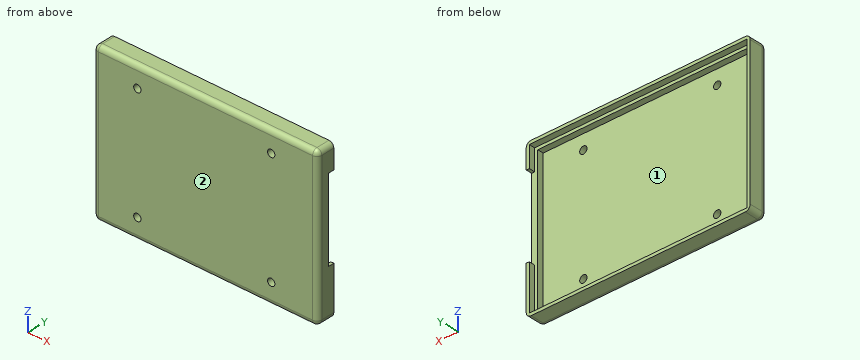
Autodesk Inventor part; units mm, degrees
ref_plane "YZ Plane" through (0, 0, 0) normal (1, 0, 0) x (0, 1, 0)
ref_plane "XZ Plane" through (0, 0, 0) normal (0, 1, 0) x (-1, 0, 0)
ref_plane "XY Plane" through (0, 0, 0) normal (0, 0, 1) x (1, 0, 0)
sketch "Sketch1" plane through (0, 0, 0) normal (0, 1, 0) x (-1, 0, 0)
  line L0 (0, 0) -> (-92, 0)
  line L1 (-92, 0) -> (-92, -64)
  line L2 (-92, -64) -> (0, -64)
  line L3 (0, -64) -> (0, 0)
  dimension "d0" = 64
  dimension "d1" = 92
extrude "Extrusion1" add sketch "Sketch1" along normal blind 7.5
sketch "Sketch2" plane through (0, 7.5, 0) normal (0, 1, 0) x (1, 0, 0)
  line L0 (2.5, 2.5) -> (89.5, 2.5)
  line L1 (89.5, 2.5) -> (89.5, 61.5)
  line L2 (89.5, 61.5) -> (2.5, 61.5)
  line L3 (2.5, 61.5) -> (2.5, 2.5)
  line L4 (0, 64) -> (0, 0)
  line L5 (0, 0) -> (92, 0)
  line L6 (92, 0) -> (92, 64)
  line L7 (92, 64) -> (0, 64)
  dimension "d4" = 2.5
  dimension "d5" = 2.5
  dimension "d6" = 2.5
  dimension "d7" = 2.5
extrude "Extrusion2" cut sketch "Sketch2" against normal blind 5 contours L3 L2 L1 L0
fillet "Fillet1" radius 2 8 edges at (0, 3.75, 0) (46, 0, 0) (92, 3.75, 0) (92, 0, -32) (92, 3.75, -64) (46, 0, -64) (0, 3.75, -64) (0, 0, -32)
sketch "Sketch3" plane through (0, 7.5, 0) normal (0, 1, 0) x (1, 0, 0)
  line L0 (1.25, 1.25) -> (90.75, 1.25)
  line L1 (90.75, 1.25) -> (90.75, 62.75)
  line L2 (90.75, 62.75) -> (1.25, 62.75)
  line L3 (1.25, 62.75) -> (1.25, 1.25)
  line L4 (0, 62) -> (0, 2)
  line L5 (2, 0) -> (90, 0)
  line L6 (92, 2) -> (92, 62)
  line L7 (90, 64) -> (2, 64)
  point P0 (0, 0)
  dimension "d11" = 1.25
  dimension "d12" = 1.25
  dimension "d13" = 1.25
  dimension "d14" = 1.25
extrude "Extrusion3" cut sketch "Sketch3" against normal blind 2.5
sketch "Sketch4" plane through (0, 2.5, 0) normal (0, 1, 0) x (1, 0, 0)
  line L0 (5, 5) -> (87, 5)
  line L1 (87, 5) -> (87, 59)
  line L2 (87, 59) -> (5, 59)
  line L3 (5, 59) -> (5, 5)
  line L4 (2.5, 2.5) -> (2.5, 61.5)
  line L5 (89.5, 2.5) -> (2.5, 2.5)
  line L6 (2.5, 61.5) -> (89.5, 61.5)
  line L7 (89.5, 61.5) -> (89.5, 2.5)
  line L8 (18, 55.5) -> (73, 55.5)
  line L9 (73, 55.5) -> (73, 8.5)
  line L10 (73, 8.5) -> (18, 8.5)
  line L11 (18, 8.5) -> (18, 55.5)
  point P0 (0, 0)
  dimension "d17" = 2.5
  dimension "d18" = 2.5
  dimension "d19" = 2.5
  dimension "d20" = 2.5
  dimension "d21" = 14
  dimension "d22" = 13
  dimension "d23" = 54
  dimension "d24" = 82
  dimension "d25" = 3.5
  dimension "d26" = 3.5
hole "Hole1" at (18, 2.5, -8.5) at (18, 2.5, -55.5) at (73, 2.5, -55.5) at (73, 2.5, -8.5) direction (0, -1, 0) diameter 3 end through all
sketch "Sketch5" plane through (92, 2, -2) normal (1, 0, 0) x (0, 0, -1)
  line L0 (8, 5.5) -> (42, 5.5)
  line L1 (42, 5.5) -> (42, 3)
  line L2 (42, 3) -> (8, 3)
  line L3 (8, 3) -> (8, 5.5)
  line L4 (0, 5.5) -> (60, 5.5)
  line L5 (0, 0) -> (0, 5.5)
  line L6 (60, 5.5) -> (60, 0)
  point P0 (-2, -2)
  dimension "d34" = 0
  dimension "d35" = 8
  dimension "d36" = 18
  dimension "d37" = 2.5
extrude "Extrusion4" cut sketch "Sketch5" against normal blind 2.5
Input: part model. Units: mm. Frame: model coordinates. Face numbers are marked on the shaded views. Coordinates: 2 decimals unless noted, no trailing zeros. Loops run counter-clockwise (first coordinate to the right, second up) from the corner with the lowest first, then second, coordinate; pieces in that order, holes last. Notation, with made-up numbers: (11, 12) - (50, 12) arc R23 ccw to (50, 31) - close; hole circle Ø6 at (-14, -3.75). An arc over 180 degrees is marked (long way). Answer in a Markdown table with one row per item. Add a question column.
Item 1: Contact query for flat-ended pins moving along their axis: P1, Ø8, axis at x = 45, z = -8.5, coming from the +Y side; P2, Ø2.5, axis at x = 73, z = -8.5, coming from the +Y side; P3, Ø0.6, axis at x = 91.5, y = 5.5, coming from the +Z side; P4, Ø1.2, axis at y = 6.5, z = -17, coming from the +X side. Output: stop coordinate, or through.
Item 2: Section query D-D on z = -45. Return the cut outline in (x, y), then the cut area to 3 significant figures.
Item 3: Line query: line 1 along Z through (x, y) = (18, 1.95); line 2 along X through (y, z) = (1.4, -8.5); line 3 along X through (y, z) = (3.25, -56). Output: solid intervals per line, ascending. Write a range as [from, to].
Item 4: Mould query, pull axis X, two halves, no side actions, for the marked faces 1 and 2. Classes: released by +X, released by -X, zero draft, split by the parting line, or undercut.
Item 5: Section query C-C on y = 6.5. Return the cut outline in (x, z), then the cut area to 3 significant figures.
Item 6: Section query B-B on z = -55.5. Return the cut outline in (x, y), then the cut area to 3 significant figures.
Item 7: Section query A-A on x = 73. Return the cut outline in (y, z), then the cut area to 3 significant figures.
Recorded:
| question | item | result |
|---|---|---|
| 1 | P1 | y = 2.5 |
| 1 | P2 | through |
| 1 | P3 | z = -0.4 |
| 1 | P4 | x = 1.25 |
| 2 | outline | (0, 2) arc R2 ccw to (2, 0) - (90, 0) arc R2 ccw to (92, 2) - (92, 7.5) - (90.75, 7.5) - (90.75, 5) - (89.5, 5) - (89.5, 2.5) - (2.5, 2.5) - (2.5, 5) - (1.25, 5) - (1.25, 7.5) - (0, 7.5) - close |
| 2 | area | 247 mm^2 |
| 3 | line 1 | [-64, -57], [-54, -10], [-7, 0] |
| 3 | line 2 | [0.09, 16.5], [19.5, 71.5], [74.5, 91.91] |
| 3 | line 3 | [0, 2.5], [89.5, 92] |
| 4 | face 1 | undercut |
| 4 | face 2 | zero draft |
| 5 | outline | (0, -62) arc R2 ccw to (2, -64) - (90, -64) arc R2 ccw to (92, -62) - (92, -44) - (90.75, -44) - (90.75, -62.75) - (1.25, -62.75) - (1.25, -1.25) - (90.75, -1.25) - (90.75, -10) - (92, -10) - (92, -2) arc R2 ccw to (90, 0) - (2, 0) arc R2 ccw to (0, -2) - close |
| 5 | area | 338 mm^2 |
| 6 | outline | (0, 2) arc R2 ccw to (2, 0) - (16.5, 0) - (16.5, 2.5) - (2.5, 2.5) - (2.5, 5) - (1.25, 5) - (1.25, 7.5) - (0, 7.5) - close; (19.5, 0) - (71.5, 0) - (71.5, 2.5) - (19.5, 2.5) - close; (74.5, 0) - (90, 0) arc R2 ccw to (92, 2) - (92, 7.5) - (90.75, 7.5) - (90.75, 5) - (89.5, 5) - (89.5, 2.5) - (74.5, 2.5) - close |
| 6 | area | 232 mm^2 |
| 7 | outline | (0, -62) arc R2 ccw to (2, -64) - (7.5, -64) - (7.5, -62.75) - (5, -62.75) - (5, -61.5) - (2.5, -61.5) - (2.5, -57) - (0, -57) - close; (0, -54) - (2.5, -54) - (2.5, -10) - (0, -10) - close; (0, -7) - (2.5, -7) - (2.5, -2.5) - (5, -2.5) - (5, -1.25) - (7.5, -1.25) - (7.5, 0) - (2, 0) arc R2 ccw to (0, -2) - close |
| 7 | area | 162 mm^2 |
